Geometry: final body of the model. Coordinates: model frame, mm. A direction names the side the tool comes from. Round coordinates to 2 decimals unless told otherwise and drop trailing zeros. Loops run counter-clockwise (first coordinate to the right, second up) from the corner with the lowest first, then second, coordinate; pieces in that order, holes last. Notation, with made-up numbers: (-16.75, -3) - (-4.75, -3) arc R34 cw to (-4.75, 30) - close; hole circle Ø10 at (24, 54.5). An arc over 180 degrees is marked (long way). Return JSON: item names as keys, results as strings. Group by question number.
1. Section D-D on x = 15.5. Return loops of the section in (y, z), and give its area (3 significant figures).
2. Set-up query: faces 4 (the face through (0, 6.35, 4)), 5 (the face through (-6.607, 3.131, -29.755)). Return all of +Z, -Z, +X, -X, +Y, -Y with unobstructed straight access to the full face (end or side cutting, diameter ignored); none if empty.
3. Draft query along X for faces 1 (the face through (13.1, 6.35, -6.3)), 2 (the face through (14.274, 11.359, -0.628)), 3 (the face through (3.1, 3.13, -0.69)). Return one class per face: +X half, -X half, draft (parallel to the pull), parting line (faces both ways), or undercut.
4. First-contact query: pin 1 Ø3 at (y, z) = (8.5, 0) entering from -X; pin 2 Ø9 at (x, z) = (-1.5, -4.5) entering from +Y; pin 3 Ø12 at (x, z) = (21, 0.5) entering from +Y. Flat tips, straight axial feed; report the tip coordinate or a pass-through.
5. Section C-C on y = 13. Return loops of the section in (x, z) (1 decimal), and give its area (3 significant figures).
6. Material intervals for probe 1 along X at (y, z) = (14, 0); probe 2 along Z at (x, y) = (0, 4.25) (3 decimals), sorted ascending.
Autodesk Inventor part; units mm, degrees
ref_plane "YZ Plane" through (0, 0, 0) normal (1, 0, 0) x (0, 1, 0)
ref_plane "XZ Plane" through (0, 0, 0) normal (0, 1, 0) x (-1, 0, 0)
ref_plane "XY Plane" through (0, 0, 0) normal (0, 0, 1) x (1, 0, 0)
sketch "Sketch1" plane through (0, 0, 0) normal (0, 1, 0) x (-1, 0, 0)
  line L0 (0, -20.0025) -> (0, 20.0025)
  line L1 (-20.0025, 0) -> (20.0025, 0)
  circle A0 centre (0, 0) radius 14.2875
  dimension "d0" = 28.575
extrude "Extrusion1" add sketch "Sketch1" along normal blind 19.05
sketch "Sketch2" plane through (0, 19.05, 0) normal (0, 1, 0) x (1, 0, 0)
  line L0 (0, 20.0025) -> (0, -20.0025)
  line L1 (20.0025, 0) -> (-20.0025, 0)
  point P0 (0, 0)
sketch "Sketch3" plane through (0, 19.05, 0) normal (0, 1, 0) x (1, 0, 0)
  point P0 (0, 0)
hole "Hole1" at (0, 19.05, 0) direction (0, -1, 0) diameter 6.35 end through all counterbore diameter 18.288 counterbore depth 12.7
chamfer "Chamfer1" distance 1.27 angle 45 1 edges at (0, 19.05, -9.144)
fillet "Fillet1" radius 2.54 1 edges at (14.2875, 19.05, 0)
sketch "Sketch4" plane through (0, 0, 0) normal (0, -1, 0) x (1, 0, 0)
  circle A0 centre (0, 0) radius 14.2875
  circle A1 centre (0, 0) radius 30.48
  dimension "d14" = 60.96
extrude "Extrusion2" add sketch "Sketch4" against normal blind 6.35
properties material "ABS, BEIGE"
Taken from the geometry:
{
 "1": {"outline": "(0, -26.24) - (6.35, -26.24) - (6.35, 26.24) - (0, 26.24) - close", "area": "333 mm2"},
 "2": {"face 4": "+Y", "face 5": "+Y, -Y"},
 "3": {"face 1": "draft", "face 2": "parting line", "face 3": "undercut"},
 "4": {"pin 1": "x = -14.29", "pin 2": "y = 17.88", "pin 3": "y = 6.35"},
 "5": {"outline": "circle Ø28.6 at (0, 0); hole circle Ø18.3 at (0, 0)", "area": "379 mm2"},
 "6": {"probe 1": "-14.29 to -9.14, 9.14 to 14.29", "probe 2": "-30.48 to -3.175, 3.175 to 30.48"}
}
